Autodesk Fusion 360 part; units mm, degrees
sketch "Sketch1" plane through (0, 0, 0) normal (0, 1, 0) x (1, 0, 0)
  line L0 (0, 0) -> (22.8, 0)
  line L1 (22.8, 0) -> (22.8, -19.85)
  line L2 (22.8, -19.85) -> (0, -19.85)
  line L3 (0, -19.85) -> (0, 0)
  dimension "d8" = 19.85
  dimension "d9" = 22.8
extrude "Extrude1" add sketch "Sketch1" along normal blind 3
sketch "Sketch2" plane through (0, 0, 0) normal (0, 1, 0) x (1, 0, 0)
  circle A0 centre (6.5, -15.16) radius 0.875
  circle A1 centre (6.5, -2.5) radius 0.875
  line L0 (0, -19.85) -> (0, 0)
  line L1 (0, 0) -> (22.8, 0)
  dimension "d3" = 1.75
  dimension "d4" = 1.75
  dimension "d5" = 12.66
  dimension "d6" = 6.5
  dimension "d7" = 2.5
sketch "Sketch4" plane through (0, 0, 0) normal (0, -1, 0) x (1, 0, 0)
  line L0 (22.8, 19.85) -> (0, 19.85)
  line L1 (0, 19.85) -> (0, 0)
  line L2 (0, 0) -> (22.8, 0)
  line L3 (22.8, 0) -> (22.8, 19.85)
  line L4 (0, 19.85) -> (4.95, 19.85)
  line L5 (4.95, 19.85) -> (4.95, 0)
  line L6 (4.95, 0) -> (0, 0)
  line L7 (0, 0) -> (0, 19.85)
  line L8 (22.8, 19.85) -> (17.85, 19.85)
  line L9 (17.85, 19.85) -> (17.85, 0)
  line L10 (17.85, 0) -> (22.8, 0)
  line L11 (22.8, 0) -> (22.8, 19.85)
  dimension "d12" = 4.95
  dimension "d13" = 4.95
extrude "Extrude3" add sketch "Sketch4" along normal blind 5.2 contours L0 L2 L3 L8 L9 L10 L11 | L0 L1 L2 L4 L5 L6 L7
sketch "Sketch5" plane through (0, 0, 19.85) normal (0, 0, 1) x (-1, 0, 0)
  line L0 (-22.8, 5.2) -> (-22.8, -3)
  line L1 (-22.8, -3) -> (0, -3)
  line L2 (0, -3) -> (0, 5.2)
  line L3 (0, 5.2) -> (-4.95, 5.2)
  line L4 (-4.95, 5.2) -> (-4.95, 0)
  line L5 (-4.95, 0) -> (-17.85, 0)
  line L6 (-17.85, 0) -> (-17.85, 5.2)
  line L7 (-17.85, 5.2) -> (-22.8, 5.2)
  line L8 (-2, 4.25) -> (-20.8, 4.25)
  line L9 (-20.8, 4.25) -> (-20.8, 2.7)
  line L10 (-20.8, 2.7) -> (-2, 2.7)
  line L11 (-2, 2.7) -> (-2, 4.25)
  dimension "d16" = 2
  dimension "d17" = 2.7
  dimension "d18" = 1.55
  dimension "d19" = 2
extrude "Extrude4" cut sketch "Sketch5" against normal blind 21 contours L4 L6 L8 L10 | L6 L8 L9 L10 | L4 L8 L10 L11
sketch "Sketch6" plane through (0, 0, 0) normal (0, -1, 0) x (1, 0, 0)
  line L0 (17.85, 0) -> (17.85, 19.85)
  line L1 (17.85, 19.85) -> (4.95, 19.85)
  line L2 (4.95, 19.85) -> (4.95, 0)
  line L3 (4.95, 0) -> (17.85, 0)
  line L4 (17.85, 19.85) -> (15.35, 19.85)
  line L5 (15.35, 19.85) -> (15.35, 0)
  line L6 (15.35, 0) -> (17.85, 0)
  line L7 (17.85, 0) -> (17.85, 19.85)
  dimension "d22" = 2.5
extrude "Extrude5" cut sketch "Sketch6" against normal blind 1.5 contours L0 L1 L3 L4 L5 L6 L7
sketch "Sketch7" plane through (17.85, 0, 0) normal (-1, 0, 0) x (0, -1, 0)
  line L0 (2.7, 0) -> (2.7, 19.85)
  line L1 (2.7, 19.85) -> (-1.5, 19.85)
  line L2 (-1.5, 19.85) -> (-1.5, 0)
  line L3 (-1.5, 0) -> (2.7, 0)
  line L4 (2.7, 19.85) -> (1, 19.85)
  line L5 (1, 19.85) -> (1, 2)
  line L6 (1, 2) -> (2.7, 2)
  line L7 (2.7, 2) -> (2.7, 19.85)
  dimension "d25" = 2.5
  dimension "d26" = 2
  dimension "d27" = 1.7
extrude "Extrude6" cut sketch "Sketch7" against normal blind 13 contours L0 L1 L4 L5 L6 L7
sketch "Sketch8" plane through (0, -5.2, 0) normal (0, -1, 0) x (1, 0, 0)
  line L0 (0, 0) -> (4.95, 0)
  line L1 (4.95, 0) -> (4.95, 19.85)
  line L2 (4.95, 19.85) -> (0, 19.85)
  line L3 (0, 19.85) -> (0, 0)
  line L4 (0, 19.85) -> (22.8, 19.85)
  line L5 (22.8, 19.85) -> (22.8, 17.85)
  line L6 (22.8, 17.85) -> (0, 17.85)
  line L7 (0, 17.85) -> (0, 19.85)
  dimension "d30" = 2
  dimension "d31" = 22.8
extrude "Extrude7" add sketch "Sketch8" against normal blind 8 contours L1 L2 L3 L4 L6 L7 | L1 L4 L5 L6
sketch "Sketch9" plane through (0, -5.2, 0) normal (0, -1, 0) x (1, 0, 0)
  line L0 (17.85, 17.85) -> (17.85, 0)
  line L1 (17.85, 0) -> (22.8, 0)
  line L2 (22.8, 0) -> (22.8, 19.85)
  line L3 (22.8, 19.85) -> (0, 19.85)
  line L4 (0, 19.85) -> (0, 0)
  line L5 (0, 0) -> (4.95, 0)
  line L6 (4.95, 0) -> (4.95, 17.85)
  line L7 (4.95, 17.85) -> (17.85, 17.85)
  line L8 (17.85, 6) -> (22.8, 6)
  line L9 (22.8, 6) -> (22.8, 12)
  line L10 (22.8, 12) -> (17.85, 12)
  line L11 (17.85, 12) -> (17.85, 6)
  dimension "d34" = 6
  dimension "d35" = 6
extrude "Extrude8" cut sketch "Sketch9" against normal blind 3 contours L0 L2 L8 L9 L10 L11
sketch "Sketch10" plane through (0, 0, 0) normal (-1, 0, 0) x (0, -1, 0)
  line L0 (5.2, 19.85) -> (-3, 19.85)
  line L1 (-3, 19.85) -> (-3, 0)
  line L2 (-3, 0) -> (5.2, 0)
  line L3 (5.2, 0) -> (5.2, 19.85)
  line L4 (-3, 11) -> (5.2, 11)
  line L5 (5.2, 11) -> (5.2, 6)
  line L6 (5.2, 6) -> (-3, 6)
  line L7 (-3, 6) -> (-3, 11)
  dimension "d38" = 5
  dimension "d39" = 6
extrude "Extrude9" add sketch "Sketch10" along normal blind 8 contours L1 L3 L4 L5 L6 L7
sketch "Sketch11" plane through (0, 0, 11) normal (0, 0, 1) x (-1, 0, 0)
  line L0 (0, 5.2) -> (0, -3)
  line L1 (0, -3) -> (8, -3)
  line L2 (8, -3) -> (8, 5.2)
  line L3 (8, 5.2) -> (0, 5.2)
  circle A0 centre (4, 1.1) radius 2.75
  dimension "d42" = 4.1
  dimension "d43" = 4
  dimension "d44" = 5.5
extrude "Extrude10" cut sketch "Sketch11" against normal blind 1 contours A0
sketch "Sketch12" plane through (0, 0, 10) normal (0, 0, 1) x (-1, 0, 0)
  circle A0 centre (4, 1.1) radius 2.75
  circle A1 centre (4, 1.1) radius 1.5
  dimension "d47" = 3
extrude "Extrude11" cut sketch "Sketch12" against normal blind 4 contours A1
sketch "Sketch13" plane through (0, 0, 0) normal (0, -1, 0) x (1, 0, 0)
  line L0 (15.35, 17.85) -> (4.95, 17.85)
  line L1 (4.95, 17.85) -> (4.95, 0)
  line L2 (4.95, 0) -> (15.35, 0)
  line L3 (15.35, 0) -> (15.35, 17.85)
  line L4 (15.35, 17.85) -> (4.95, 17.85)
  line L5 (4.95, 17.85) -> (4.95, 0)
  line L6 (4.95, 0) -> (15.35, 0)
  line L7 (15.35, 0) -> (15.35, 17.85)
extrude "Extrude12" cut sketch "Sketch13" against normal blind 0.1
equation "d14 = 2.5 mm + 2.7 mm"
Model file for the job. Use its own axes, mm. A direction names the side the tool comes from. Coordinates: 2 decimals unless noted, no trailing zeros. Order: outer loops, then holes, each group sorted by start corner. A loop starts at its lowest first (then second) coordinate and runs counter-clockwise, first axis right, second up. Notation, with made-up numbers: (-4, 82) -> (51, 82) arc R8 cw to (51, 86) -> close; hole circle Ø2 at (-4.5, -26). An arc over 180 degrees is marked (long way). Answer as a JSON object with one key per item and string values. Group by question number.
1) Which spindle directions (+Z, -Z, +X, -X, +Y, -Y) get a long thin tool onto all of the face, cutting with end or side? Do faces 4 (the face through (3, -2.7, 9)), 5 (the face through (-6, -1, 6)), 6 (the face through (0, -1, 15)), 7 (the face through (4.95, -1, 9)). Say none if no direction does.
2) Cut at C-C, the plane y = -1.75. Write the cut outline in (x, z), then the cut area to 3 significant figures.
3) Flat gauge pins, fed straight in: pin 1 (2.5 mm diameter, centred on x = -4.5, y = -1.5, fed in from +Z); pin 2 (1.5 mm diameter, centred on x = 9, y = -1.5, fed in from -Z); pin 3 (3 mm diameter, centred on x = 11, z = 4.5, fed in from -Y). Where does each tip first touch, or does it go through?
4) Cut at B-B, the plane y = -0.25. Write the cut outline in (x, z).
5) Cut at A-A, the plane x = -3. Write the cut outline in (y, z).
6) Drill centre lines: L1, parallel to Y at x = -4, z = 7.05; L2, parallel to Y at x = -4, z = 10.6; L3, parallel to X at y = 0, z = 12.75. Where is each one in solid material? Low to high.
7) Cut at D-D, the plane x = 4.5. Write the cut outline in (y, z).
8) Pull direction Z, two halves, no side cores. Call faces 1 (the face through (-5.2, 0.1, 10)), 2 (the face through (20, -1, 10)), 3 (the face through (-3.404, 1.585, 10.507)): +Z half, -Z half, draft (parallel to the pull), parting line (faces both ways), or undercut.
Check values:
{
 "1": {"face 4": "-Z", "face 5": "-Z, -X, +Y, -Y", "face 6": "+Z, -X, +Y, -Y", "face 7": "-Z, -Y"},
 "2": {"outline": "(-8, 6) -> (-5.35, 6) -> (-5.35, 10) -> (-6.67, 10) -> (-6.67, 11) -> (-8, 11) -> close; (-2.65, 6) -> (0, 6) -> (0, 0) -> (4.95, 0) -> (4.95, 17.85) -> (22.8, 17.85) -> (22.8, 19.85) -> (0, 19.85) -> (0, 11) -> (-1.33, 11) -> (-1.33, 10) -> (-2.65, 10) -> close; (17.85, 0) -> (22.8, 0) -> (22.8, 2) -> (17.85, 2) -> close", "area": "168 mm²"},
 "3": {"pin 1": "stops at z = 10", "pin 2": "stops at z = 17.85", "pin 3": "stops at y = 0.1"},
 "4": {"outline": "(-8, 6) -> (-5.24, 6) -> (-5.24, 10) -> (-6.62, 10) -> (-6.62, 11) -> (-8, 11) -> close; (-2.76, 6) -> (0, 6) -> (0, 0) -> (4.95, 0) -> (4.95, 17.85) -> (17.85, 17.85) -> (17.85, 0) -> (22.8, 0) -> (22.8, 19.85) -> (0, 19.85) -> (0, 11) -> (-1.38, 11) -> (-1.38, 10) -> (-2.76, 10) -> close"},
 "5": {"outline": "(-5.2, 6) -> (-2.22, 6) -> (-2.22, 10) -> (-3.66, 10) -> (-3.66, 11) -> (-5.2, 11) -> close; (0.02, 6) -> (3, 6) -> (3, 11) -> (1.46, 11) -> (1.46, 10) -> (0.02, 10) -> close"},
 "6": {"L1": "y = -5.2 to -2.6, 0.4 to 3", "L2": "y = -5.2 to -3.85, 1.65 to 3", "L3": "x = 0 to 4.95, 17.85 to 22.8"},
 "7": {"outline": "(-5.2, 0) -> (-4.25, 0) -> (-4.25, 17.85) -> (-2.7, 17.85) -> (-2.7, 0) -> (3, 0) -> (3, 19.85) -> (-5.2, 19.85) -> close"},
 "8": {"face 1": "+Z half", "face 2": "undercut", "face 3": "draft"}
}
